Build history of the part. All positions in model axes, mm. A direction names the side the tool comes from. Round coordinates to 2 decimals unless told otherwise and drop trailing zeros. Write each loop counter-clockwise with the first axis right and the second up, starting at its lowest first coordinate (ties: lowest second). Pieces come first, ordered by that corner, then holes.
1) Saw through at B-B (x = 210.5). Write the cut outline in (y, z), plus the area to 3 significant figures.
2) Flat gauge pins, fed straight in: pin 1 (15 mm diameter, centred on x = 300, z = 42.5, fed in from -Y); pin 2 (6 mm diameter, centred on x = 321, z = 38, fed in from +Y); pin 3 (13.5 mm diameter, centred on x = 306.5, y = 132, fed in from -Z). Where does each tip first touch, or does it go through?
3) Which spindle directions (+Z, -Z, +X, -X, +Y, -Y) get a long thin tool onto all of the face, cutting with end or side? Do faces 1 (the flat face through (300, 100, 20)), 2 (the flat face through (300, 70, 35)), 3 (the flat face through (171.03, 487.88, 5.07)), 4 (the flat face through (275, 99, 40)), 5 (the flat face through (300, 123, 40)). Say none if no direction does.
4) Saw through at C-C (y = 84). Write the cut outline in (x, z), plus the area to 3 significant figures.
5) Saw through at A-A (y = 366). Write the cut outline in (x, z).
6) Saw through at D-D (y = 562). Write the cut outline in (x, z).
7) Wall check: probe 1 along X at (y, z) = (125.5, 4); probe 2 along Z at (x, y) = (506, 133); probe 3 along Y at (x, z) = (165.5, 4). Give the ranges that are in metal, low to high.
8) Pull direction Y, two halves, no side cores. Call faces 6 (the flat face through (213.79, 333.69, 5.07)), 7 (the flat face through (300, 145, 50)), 8 (the flat face through (325, 99, 40)): +Y half, -Y half, draft (parallel to the pull), parting line (faces both ways), or undercut.
Autodesk Inventor part; units mm, degrees
ref_plane "YZ Plane" through (0, 0, 0) normal (1, 0, 0) x (0, 1, 0)
ref_plane "XZ Plane" through (0, 0, 0) normal (0, 1, 0) x (-1, 0, 0)
ref_plane "XY Plane" through (0, 0, 0) normal (0, 0, 1) x (1, 0, 0)
sketch "Sketch1" plane through (0, 0, 0) normal (0, 0, 1) x (1, 0, 0)
  line L0 (0, 0) -> (600, 0)
  line L1 (600, 0) -> (600, 600)
  line L2 (600, 600) -> (0, 600)
  line L3 (0, 600) -> (0, 0)
  dimension "d0" = 600
  dimension "d1" = 600
extrude "Extrusion1" add sketch "Sketch1" along normal blind 10
sketch "Sketch2" plane through (0, 0, 10) normal (0, 0, 1) x (1, 0, 0)
  line L0 (193.5, 368) -> (406.5, 368)
  line L1 (406.5, 368) -> (406.5, 481)
  line L2 (406.5, 481) -> (193.5, 481)
  line L3 (193.5, 481) -> (193.5, 368)
  line L4 (0, 600) -> (0, 0)
  line L5 (600, 600) -> (0, 600)
  dimension "d4" = 213
  dimension "d5" = 113
  dimension "d6" = 193.5
  dimension "d7" = 119
extrude "Extrusion2" cut sketch "Sketch2" against normal through all
sketch "Sketch3" plane through (0, 0, 10) normal (0, 0, 1) x (1, 0, 0)
  circle A0 centre (144.1129, 397.844) radius 80 construction
  circle A1 centre (455.8871, 397.844) radius 80 construction
  line L0 (220, 501) -> (380, 501)
  line L1 (380, 501) -> (338.589, 346.4519) construction
  line L2 (220, 501) -> (261.411, 346.4519) construction
  line L3 (261.411, 346.4519) -> (338.589, 346.4519)
  line L4 (123.4074, 475.1181) -> (220, 501)
  line L5 (261.411, 346.4519) -> (164.8185, 320.57)
  arc A2 (123.4074, 475.1181) -> (164.8185, 320.57) centre (144.1129, 397.844) ccw
  line L6 (380, 501) -> (476.5926, 475.1181)
  line L7 (338.589, 346.4519) -> (435.1815, 320.57)
  arc A3 (435.1815, 320.57) -> (476.5926, 475.1181) centre (455.8871, 397.844) ccw
  line L8 (193.5, 481) -> (406.5, 481)
  point P0 (0, 0)
  point P1 (424.4703, 324.271)
  point P2 (300, 481)
  point P3 (300, 501)
  dimension "d10" = 160
  dimension "d11" = 160
  dimension "d12" = 160
  dimension "d13" = 160
  dimension "d14" = 160
  dimension "d15" = 75
  dimension "d16" = 75
  dimension "d17" = 100
  dimension "d18" = 100
  dimension "d19" = 20
extrude "Extrusion3" cut sketch "Sketch3" against normal through all
sketch "Sketch4" plane through (0, 0, 10) normal (0, 0, 1) x (1, 0, 0)
  line L0 (275, 150) -> (325, 150)
  line L1 (325, 150) -> (325, 100)
  line L2 (325, 100) -> (275, 100)
  line L3 (275, 100) -> (275, 150)
  line L4 (0, 0) -> (600, 0)
  point P0 (300, 100)
  point P1 (300, 0)
  dimension "d22" = 50
  dimension "d23" = 50
  dimension "d24" = 100
extrude "Extrusion4" cut sketch "Sketch4" against normal through all
sketch "Sketch5" plane through (0, 0, 10) normal (0, 0, 1) x (1, 0, 0)
  line L0 (275, 100) -> (325, 100)
  line L1 (325, 100) -> (325, 70)
  line L2 (325, 70) -> (275, 70)
  line L3 (275, 70) -> (275, 100)
  point P0 (0, 0)
  dimension "d27" = 50
  dimension "d28" = 30
extrude "Extrusion5" add sketch "Sketch5" along normal blind 30
sketch "Sketch6" plane through (0, 0, 40) normal (0, 0, 1) x (1, 0, 0)
  line L0 (275, 70) -> (275, 100)
  line L1 (275, 70) -> (325, 70)
  line L2 (325, 70) -> (325, 145)
  line L3 (325, 145) -> (275, 145)
  line L4 (275, 145) -> (275, 70)
  point P0 (0, 0)
  dimension "d31" = 50
  dimension "d32" = 75
extrude "Extrusion6" add sketch "Sketch6" along normal blind 20
properties part number "Top Cover" material "ABS Plastic"
Evaluation:
1. outline: (0, 0) - (332.81, 0) - (332.81, 10) - (0, 10) - close; (498.45, 0) - (600, 0) - (600, 10) - (498.45, 10) - close
1. area: 4,340 mm2
2. pin 1: stops at y = 70
2. pin 2: stops at y = 145
2. pin 3: stops at z = 40
3. face 1: -Z
3. face 2: +Z, +X, -X, -Y
3. face 3: +Z, -Z
3. face 4: +Z, -X, +Y, -Y
3. face 5: -Z, +X, -X, +Y
4. outline: (0, 0) - (600, 0) - (600, 10) - (325, 10) - (325, 60) - (275, 60) - (275, 10) - (0, 10) - close
4. area: 8,500 mm2
5. outline: (0, 0) - (70.72, 0) - (70.72, 10) - (0, 10) - close; (529.28, 0) - (600, 0) - (600, 10) - (529.28, 10) - close
6. outline: (0, 0) - (600, 0) - (600, 10) - (0, 10) - close
7. probe 1: x = 0 to 275, 325 to 600
7. probe 2: z = 0 to 10
7. probe 3: y = 0 to 320.75, 486.4 to 600
8. face 6: undercut
8. face 7: +Y half
8. face 8: draft
